from build123d import *

# Parameters (mm, degrees)
SKETCH1_R           = 1
SKETCH1_W           = 10
SKETCH1_H           = 3
SKETCH1_R_2         = 0.5
SKETCH1_R_3         = 0.5706303
BOSS_EXTRUDE1_DEPTH = 2
SKETCH1_3_W         = 5
SKETCH1_3_H         = 5
BOSS_EXTRUDE2_DEPTH = 5
SKETCH1_4_W         = 10
SKETCH1_4_H         = 3
BOSS_EXTRUDE3_DEPTH = 3


with BuildPart() as part:
    # Sketch1 → Boss-Extrude1 (new body)
    with BuildSketch(Plane.XY):
        Polygon((3.5, 7.35633001), (-16.2, 7.35633001), (-16.2, -8.64366999), (-11.2, -8.64366999), (-1.5, -8.64366999), (3.5, -8.64366999), (3.5, -1.64366999), (-1.5, -1.64366999), (-1.5, 3.35633001), (3.5, 3.35633001), align=None)
        with Locations((-14.2, -6.64366999)):
            Circle(SKETCH1_R, mode=Mode.SUBTRACT)
        with Locations((-7.2, -1.5)):
            Rectangle(SKETCH1_W, SKETCH1_H, mode=Mode.SUBTRACT)
        with Locations((1.5, -6.64366999)):
            Circle(SKETCH1_R, mode=Mode.SUBTRACT)
        with Locations((-14.2, 5.35633001)):
            Circle(SKETCH1_R, mode=Mode.SUBTRACT)
        with Locations((-11, 5.35633001)):
            Circle(SKETCH1_R_2, mode=Mode.SUBTRACT)
        with Locations((-9.5, 5.35633001)):
            Circle(SKETCH1_R_3, mode=Mode.SUBTRACT)
        with Locations((-8, 5.35633001)):
            Circle(SKETCH1_R_2, mode=Mode.SUBTRACT)
        with Locations((-6.5, 5.35633001)):
            Circle(SKETCH1_R_2, mode=Mode.SUBTRACT)
        with Locations((-5, 5.35633001)):
            Circle(SKETCH1_R_3, mode=Mode.SUBTRACT)
        with Locations((-3.5, 5.35633001)):
            Circle(SKETCH1_R_2, mode=Mode.SUBTRACT)
        with Locations((1.5, 5.35633001)):
            Circle(SKETCH1_R, mode=Mode.SUBTRACT)
    extrude(amount=BOSS_EXTRUDE1_DEPTH)

    # Sketch1<3> → Boss-Extrude2 (add)
    with BuildSketch(Plane.XY):
        with Locations((1, 0.85633001)):
            Rectangle(SKETCH1_3_W, SKETCH1_3_H)
    extrude(amount=BOSS_EXTRUDE2_DEPTH)

    # Sketch1<4> → Boss-Extrude3 (add)
    with BuildSketch(Plane.XY):
        with Locations((-7.2, -1.5)):
            Rectangle(SKETCH1_4_W, SKETCH1_4_H)
    extrude(amount=BOSS_EXTRUDE3_DEPTH)


solid = part.part
For this review, take the finished solid that the model builds, in its own axes (mm). A direction names the side the tool comes from. Round coordinates to 2 decimals unless told otherwise and drop trailing zeros. Loops run counter-clockwise (first coordinate to the right, second up) from the corner with the lowest first, then second, coordinate; pieces in that order, holes last. Notation, with made-up numbers: (-26.75, 81.25) - (29.25, 81.25) arc R31 cw to (29.25, 107.25) - close; hole circle Ø1 at (-9, -14.5). An arc over 180 degrees is marked (long way). Use one line per item in the form item = value.
1) Clearance check with flat-ended pins moving along their axes: P1, Ø2.5, axis at x = 1.5, y = -6.64, coming from the +Z side; P2, Ø0.5, axis at y = -1.5, z = 2.5, coming from the -X side; P3, Ø8, axis at x = -10.5, y = 1, coming from the +Z side; P4, Ø2.5, axis at x = -14.2, y = -6.64, coming from the -Z side. State where each tip first meets the part, or that it passes through.
Solutions:
P1 = 2
P2 = -12.2
P3 = 3
P4 = 0
2) We need section D-D on x = -6.5. Write out the cut boundary in (y, z).
Solutions:
outline = (-8.64, 0) - (4.86, 0) - (4.86, 2) - (0, 2) - (0, 3) - (-3, 3) - (-3, 2) - (-8.64, 2) - close; (5.86, 0) - (7.36, 0) - (7.36, 2) - (5.86, 2) - close
3) We need section C-C on z = 0.45. State how many separate pieces and enclosed holes the cut face has, then the cut area to 3 significant figures.
Solutions:
separate_pieces = 1
enclosed_holes = 10
area = 297 mm2
4) We need section B-B on x = 1.5. Write out the cut boundary in (y, z), then the cut area to 3 significant figures.
Solutions:
outline = (-8.64, 0) - (-7.64, 0) - (-7.64, 2) - (-8.64, 2) - close; (-5.64, 0) - (4.36, 0) - (4.36, 2) - (3.36, 2) - (3.36, 5) - (-1.64, 5) - (-1.64, 2) - (-5.64, 2) - close; (6.36, 0) - (7.36, 0) - (7.36, 2) - (6.36, 2) - close
area = 39.0 mm2
5) Tool access review of faces 4 (the face through (1, 3.356, 3)), 5 (the face through (1, -1.644, 3)), 6 (the face through (-16.2, -1, 1)), 7 (the face through (-7, -1, 3)), 8 (the face through (-13.246, 5.657, 0.986)): name each direction out of +Z, -Z, +X, -X, +Y, -Y from which nothing blocks a thin tool from reaching the whole face with its end or side.
Solutions:
face_4 = +Z, +X, -X, +Y
face_5 = +Z, +X, -Y
face_6 = +Z, -Z, -X, +Y, -Y
face_7 = +Z, -X, +Y, -Y
face_8 = +Z, -Z
6) Mouldability with a two-part tool opening along Y and no side actions: class faces 1 (the face through (-6, -8.644, 1)), 2 (the face through (-2.2, -1.5, 2.5)), 3 (the face through (-7.523, 5.507, 0.986)) as pulls with the +Y half, pulls with the -Y half, needs draft (parallel to the pull), parting line crosses it, or undercut.
Solutions:
face_1 = pulls with the -Y half
face_2 = needs draft
face_3 = undercut
7) We need section A-A on x = -9.5. Write out the cut boundary in (y, z).
Solutions:
outline = (-8.64, 0) - (4.79, 0) - (4.79, 2) - (0, 2) - (0, 3) - (-3, 3) - (-3, 2) - (-8.64, 2) - close; (5.93, 0) - (7.36, 0) - (7.36, 2) - (5.93, 2) - close
8) Wall thickness on probe 1 along Y at (x, z) = (-14.2, 0.85); probe 2 along Y at (x, z) = (-6.5, 0.8); probe 3 along Z at (x, y) = (0.25, -3): over which ranges is each line inside the solid? List them lowest first.
Solutions:
probe_1 = -8.64 to -7.64, -5.64 to 4.36, 6.36 to 7.36
probe_2 = -8.64 to 4.86, 5.86 to 7.36
probe_3 = 0 to 2
